Verification items for this drawing (mm, ordinates from the low corner). A direction names the side the tool comes from. Give positions to 0.01 mm unless a question says otherwise; leave off trailing zeros. Write each loop counter-clockwise with the first axis right and the second up, starting at its lowest first coordinate (ties: lowest second). Pieces come first, ordered by that corner, then holes. Notation, with made-up numbers: (59.5, 28.25) -> (65.5, 28.25) arc R16 cw to (65.5, 59.25) -> close; hole circle Ø4 at (39, -27.75). An arc over 180 degrees is marked (long way). Answer as a JSON object with one key per item and string values.
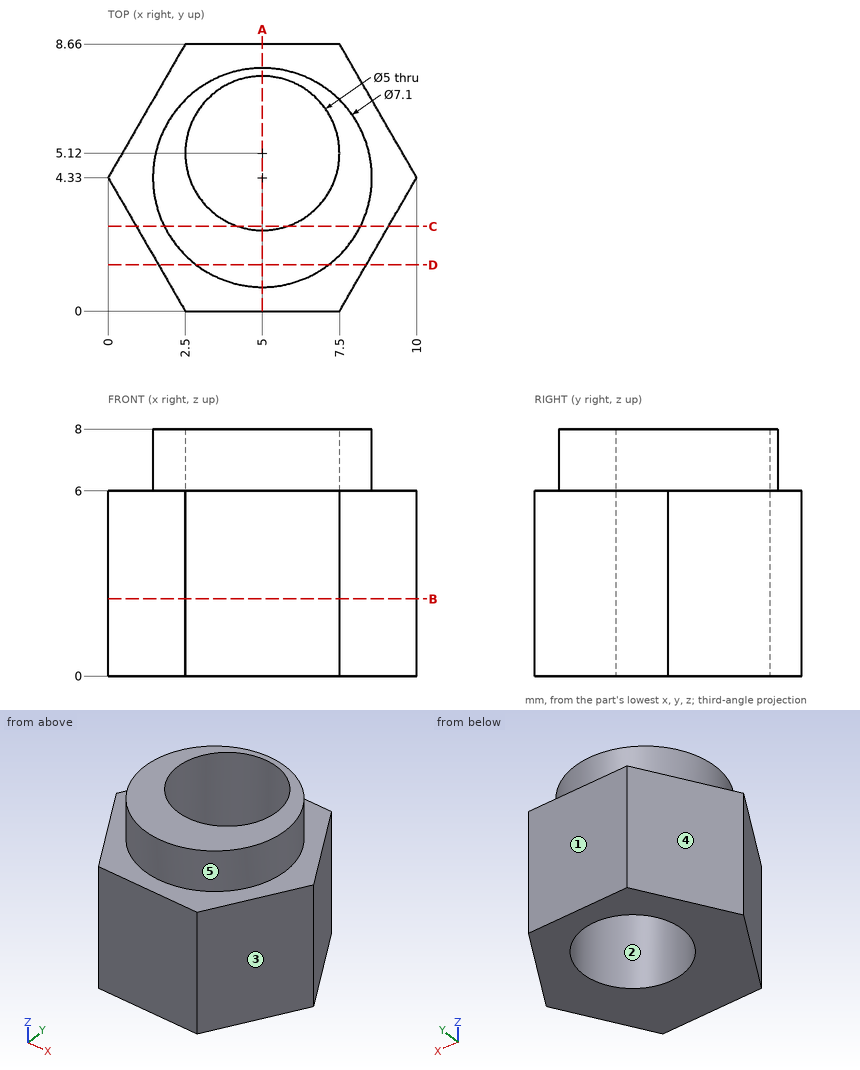
1. Go/stop test with flat-tipped pins: P1, Ø1.5, axis at y = 3, z = 4.5, coming from the -X side (1 decimal); P2, Ø2, axis at y = 3.5, z = 5, coming from the -X side. Record where each tip stops, or that it passes through.
Determined:
{"P1": "x = 0.3", "P2": "x = 0"}
2. Scan lines: L1, parallel to Y at x = 5, z = 6.5; L2, parallel to X at y = 3.25, z = 5.5 (1 decimal); L3, parallel to Y at x = 5, z = 5. Record each from-to range of solid material in increasing order. Write a range as [from, to].
Determined:
{"L1": "[0.78, 2.62], [7.62, 7.88]", "L2": "[0.6, 3.3], [6.7, 9.4]", "L3": "[0, 2.62], [7.62, 8.66]"}
3. Access from +Z, -Z, +X, -X, +Y, -Y to the whole of each face (thin tool, end or side, straight path). Record for the marked faces 4 and 5.
Determined:
{"face 4": "+Z, -Z, -X, +Y", "face 5": "+Z"}
4. Sectioned sample at D-D, the plane y = 1.5. Enter the section's corners in (x, z).
Determined:
{"outline": "(1.63, 0) -> (8.37, 0) -> (8.37, 6) -> (7.14, 6) -> (7.14, 8) -> (2.86, 8) -> (2.86, 6) -> (1.63, 6) -> close"}
5. Mould release check, pull along X, two halves, no side actions. Record for the marked faces 1, 2 and 3: released by +X, released by -X, zero draft, split by the parting line, or undercut.
Determined:
{"face 1": "zero draft", "face 2": "undercut", "face 3": "released by +X"}
6. Sectioned sample at C-C, the plane y = 2.75. Enter the section's corners in (x, z) (1 decimal).
Determined:
{"outline": "(0.9, 0) -> (4.2, 0) -> (4.2, 8) -> (1.8, 8) -> (1.8, 6) -> (0.9, 6) -> close; (5.8, 0) -> (9.1, 0) -> (9.1, 6) -> (8.2, 6) -> (8.2, 8) -> (5.8, 8) -> close"}
7. Sectioned sample at A-A, the plane x = 5. Enter the section's corners in (y, z).
Determined:
{"outline": "(0, 0) -> (2.62, 0) -> (2.62, 8) -> (0.78, 8) -> (0.78, 6) -> (0, 6) -> close; (7.62, 0) -> (8.66, 0) -> (8.66, 6) -> (7.88, 6) -> (7.88, 8) -> (7.62, 8) -> close"}
8. Sectioned sample at B-B, the plane z = 2.5. Enter the section's corners in (x, y).
Determined:
{"outline": "(0, 4.33) -> (2.5, 0) -> (7.5, 0) -> (10, 4.33) -> (7.5, 8.66) -> (2.5, 8.66) -> close; hole circle Ø5 at (5, 5.12)"}
